Could you check a few things on this model? Use its own coordinates, in mm. Face numbers are marked on the shaded views. A direction names the side the tool comes from. Round coordinates to 2 decimals unless told otherwise and drop trailing zeros. Loops run counter-clockwise (first coordinate to the right, second up) from the corner with the lowest first, then second, coordinate; pieces in that order, holes last. Notation, with made-up numbers: M -25.75,7.25 L 13.25,7.25 A9 ccw 13.25,20.25 Z; hole C 49,48.5 d4. An arc over 180 degrees is marked long. Answer in a Markdown table with one row per item.
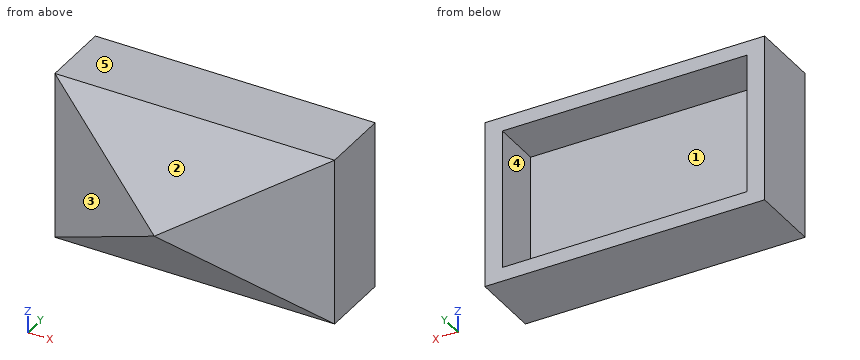
```python
from build123d import *

# Parameters (mm, degrees)
SKETCH2_W           = 40
SKETCH2_H           = 24
BOSS_EXTRUDE1_DEPTH = 10
SKETCH3_W           = 35
SKETCH3_H           = 20
CUT_EXTRUDE1_DEPTH  = 7


with BuildPart() as part:
    # Sketch2 → Boss-Extrude1 (new body)
    with BuildSketch(Plane(origin=(0, 0, 0), x_dir=(1, 0, 0), z_dir=(0, 1, 0))):
        Rectangle(SKETCH2_W, SKETCH2_H)
    extrude(amount=BOSS_EXTRUDE1_DEPTH)

    # Sketch3 → Cut-Extrude1 (cut)
    with BuildSketch(Plane(origin=(0, 10, 0), x_dir=(1, 0, 0), z_dir=(0, 1, 0))):
        Rectangle(SKETCH3_W, SKETCH3_H)
    extrude(amount=-CUT_EXTRUDE1_DEPTH, mode=Mode.SUBTRACT)

    # Sketch9 → Loft1 section 0
    with BuildSketch(Plane.XZ, mode=Mode.PRIVATE) as loft1_s0:
        with BuildLine():
            Line((20, -12), (-20, -12))
            Line((-20, -12), (-20, 12))
            Line((-20, 12), (20, 12))
            Line((20, 12), (20, -12))
        make_face()
    loft([loft1_s0.sketch, Vertex(0, -10, 0)])


solid = part.part
```
1) Which directions (+Z, -Z, +X, -X, +Y, -Y) give clear straight access to the entire face, cutting with the end or side of a thin tool? Please do the marked faces 4 and 5.
Computed:
| item | result |
|---|---|
| face 4 | +Y |
| face 5 | +Z, +X, -X, +Y, -Y |
2) If we mould it in two halves opening along X, with no side actions, what happens to the marked faces 1, 2 and 3? For each: released by +X, released by -X, zero draft, split by the parting line, or undercut.
Computed:
| item | result |
|---|---|
| face 1 | undercut |
| face 2 | zero draft |
| face 3 | released by -X |
3) I want a section at A-A, the plane x = -15. Please give me the cut outline in (y, z), plus the area to 4 significant figures.
Computed:
| item | result |
|---|---|
| outline | M -2.5,-9 L 0,-12 L 10,-12 L 10,-10 L 3,-10 L 3,10 L 10,10 L 10,12 L 0,12 L -2.5,9 Z |
| area | 152.5 mm² |
4) I need wall thicknesses on line 1 (X direction, y = 3.5, z = -9); line 2 (Z direction, x = 7.5, y = 3.25); line 3 (X direction, y = -5, z = 5.25). Which ranges of each line are inside material? Lowest first, please.
Computed:
| item | result |
|---|---|
| line 1 | x = -20 to -17.5, 17.5 to 20 |
| line 2 | z = -12 to -10, 10 to 12 |
| line 3 | x = -10 to 10 |
5) I want a section at B-B, the plane y = 4. Please give me the cut outline in (x, z), plus the area to 3 significant figures.
Computed:
| item | result |
|---|---|
| outline | M -20,-12 L 20,-12 L 20,12 L -20,12 Z; hole M -17.5,-10 L 17.5,-10 L 17.5,10 L -17.5,10 Z |
| area | 260 mm² |
6) I want a section at C-C, the plane z = -6.75. Please give me the cut outline in (x, y) (3 decimals).
Computed:
| item | result |
|---|---|
| outline | M -20,0 L -11.25,-4.375 L 11.25,-4.375 L 20,0 L 20,10 L 17.5,10 L 17.5,3 L -17.5,3 L -17.5,10 L -20,10 Z |
7) Will these pins go through, and if not, where does the flat tip stop? P1, Ø1, axis at y = -6, z = 1.5, coming from the -X side; P2, Ø1.5, axis at y = -2.5, z = 5.5, coming from the -X side; P3, Ø4, axis at x = 11.5, y = -4, coming from the +Z side.
Computed:
| item | result |
|---|---|
| P1 | stops at x = -9 |
| P2 | stops at x = -16.5 |
| P3 | stops at z = 9.6 |
8) I want a section at D-D, the plane y = -6.25. Please give me the cut outline in (x, z).
Computed:
| item | result |
|---|---|
| outline | M -7.5,-4.5 L 7.5,-4.5 L 7.5,4.5 L -7.5,4.5 Z |
